from build123d import *

# Parameters (mm, degrees)
SKETCH_1_W           = 2.5
SKETCH_1_H           = 2
EXTRUDE_1_DEPTH      = 5
EXTRUDE_3_DEPTH      = 1
EXTRUDE_3_DEPTH_BACK = 1
SKETCH_2_W           = 4.5
SKETCH_2_H           = 4
SKETCH_2_W_2         = 2.5
SKETCH_2_H_2         = 2


with BuildPart() as part:
    # 草图1 → 凸台-拉伸1 (new body)
    with BuildSketch(Plane.XY):
        with Locations((1.25, 1)):
            Rectangle(SKETCH_1_W, SKETCH_1_H)
    extrude(amount=EXTRUDE_1_DEPTH)

    # 草图2 → 凸台-拉伸3 (add, two sides: drawn at the far end of the back side and taken through both)
    with BuildSketch(Plane(origin=(0, 0, 0), x_dir=(-1, 0, 0), z_dir=(0, 0, -1)).offset(-EXTRUDE_3_DEPTH_BACK)):
        with Locations((-1.25, 1)):
            Rectangle(SKETCH_2_W, SKETCH_2_H)
        with Locations((-1.25, 1)):
            Rectangle(SKETCH_2_W_2, SKETCH_2_H_2, mode=Mode.SUBTRACT)
    extrude(amount=EXTRUDE_3_DEPTH + EXTRUDE_3_DEPTH_BACK)


solid = part.part
Model file for the job. Use its own axes, mm. A direction names the side the tool comes from. Coordinates: 2 decimals unless noted, no trailing zeros. Loops run counter-clockwise (first coordinate to the right, second up) from the corner with the lowest first, then second, coordinate; pieces in that order, holes last. Notation, with made-up numbers: (-7.75, 87) -> (8.25, 87) arc R38 cw to (8.25, 125) -> close; hole circle Ø9 at (-35.75, -22.75). An arc over 180 degrees is marked (long way). Use one line per item in the form item = value. Start each with the question number.
(1) Probe probe 1 along X at (y, z) = (0.1, -0.7); probe 2 along Y at (x, z) = (1.5, -0.1); probe 3 along X at (y, z) = (0.5, 3.1). List the from-to ranges inside material, lowest first. Write a range as from..to.
(2) Tool access for faces 1 (the flat face through (2.5, 1, 3)), 2 (the flat face through (2.5, 1, -0.5)), 3 (the flat face through (0, 1, 3)): list every direction of +Z, -Z, +X, -X, +Y, -Y with a clear straight run to the whole face (end or side of a thin tool).
(3) Cut at C-C on z = 2.55. Give the cut face in (x, y), and give its area (3 significant figures).
(4) Cut at D-D on x = 2.8. Give the cut face in (y, z), and give its area (3 significant figures).
(5) Flat gauge pins, fed straight in: pin 1 (1 mm diameter, centred on x = 2, z = 2, fed in from -Y); pin 2 (1.2 mm diameter, centred on x = 1.5, z = 2.5, fed in from +Y); pin 3 (1.6 mm diameter, centred on y = 0.5, z = 3, fed in from -X). Where does each tip first touch, or does it go through?
(6) Pull direction Y, two halves, no side cores. Call faces 4 (the flat face through (1, 0, 3)), 5 (the flat face through (-1, 1, 0)), 6 (the flat face through (0, 1, -0.5)): pulls with the +Y half, pulls with the -Y half, needs draft (parallel to the pull), parting line crosses it, or undercut.
(7) Cut at B-B on x = 1. Give the cut face in (y, z).
(8) Cut at A-A on y = 0.6. Give the cut face in (x, z), and give its area (3 significant figures).
Values:
q1.probe_1 = -1..0, 2.5..3.5
q1.probe_2 = -1..0, 2..3
q1.probe_3 = 0..2.5
q2.face_1 = +Z, +X, +Y, -Y
q2.face_2 = -Z
q2.face_3 = +Z, -X, +Y, -Y
q3.outline = (0, 0) -> (2.5, 0) -> (2.5, 2) -> (0, 2) -> close
q3.area = 5.00 mm2
q4.outline = (-1, -1) -> (3, -1) -> (3, 1) -> (-1, 1) -> close
q4.area = 8.00 mm2
q5.pin_1 = 0
q5.pin_2 = 2
q5.pin_3 = 0
q6.face_4 = pulls with the -Y half
q6.face_5 = needs draft
q6.face_6 = undercut
q7.outline = (-1, -1) -> (0, -1) -> (0, 0) -> (2, 0) -> (2, -1) -> (3, -1) -> (3, 1) -> (2, 1) -> (2, 5) -> (0, 5) -> (0, 1) -> (-1, 1) -> close
q8.outline = (-1, -1) -> (0, -1) -> (0, 0) -> (2.5, 0) -> (2.5, -1) -> (3.5, -1) -> (3.5, 1) -> (2.5, 1) -> (2.5, 5) -> (0, 5) -> (0, 1) -> (-1, 1) -> close
q8.area = 16.5 mm2
